from build123d import *

# Parameters (mm, degrees)
BOSS_EXTRUDE1_DEPTH = 7.62
SKETCH2_R           = 7.112
SKETCH2_R_2         = 3.81
BOSS_EXTRUDE2_DEPTH = 12.7
CHAMFER1_SIZE       = 0.508


with BuildPart() as part:
    # Sketch1 → Boss-Extrude1 (new body)
    with BuildSketch(Plane(origin=(0, 0, 0), x_dir=(1, 0, 0), z_dir=(0, 1, 0))):
        Polygon((9.144, 2.794), (7.112, 2.794), (7.112, -2.794), (9.144, -2.794), (9.144, -9.144), (2.794, -9.144), (2.794, -7.112), (-2.794, -7.112), (-2.794, -9.144), (-9.144, -9.144), (-9.144, -2.794), (-7.112, -2.794), (-7.112, 2.794), (-9.144, 2.794), (-9.144, 9.144), (-2.794, 9.144), (-2.794, 7.112), (2.794, 7.112), (2.794, 9.144), (9.144, 9.144), align=None)
    extrude(amount=BOSS_EXTRUDE1_DEPTH)

    # Sketch2 → Boss-Extrude2 (add)
    with BuildSketch(Plane(origin=(0, 7.62, 0), x_dir=(1, 0, 0), z_dir=(0, 1, 0))):
        with Locations(Location((0, 0, 0), (0, 0, 270))):
            Circle(SKETCH2_R)
        with Locations(Location((0, 0, 0), (0, 0, 270))):
            Circle(SKETCH2_R_2, mode=Mode.SUBTRACT)
    extrude(amount=BOSS_EXTRUDE2_DEPTH)

    # Chamfer1
    chamfer1_edges = [part.edges().sort_by_distance(p)[0] for p in [
        (0, 20.32, -3.81),
    ]]
    chamfer(chamfer1_edges, length=CHAMFER1_SIZE)


solid = part.part
Here's how the part is built. I have some questions about the finished solid (model axes, mm). A direction names the side the tool comes from. Coordinates: 2 decimals unless noted, no trailing zeros. Write each loop counter-clockwise with the first axis right and the second up, starting at its lowest first coordinate (ties: lowest second). Pieces come first, ordered by that corner, then holes. Notation, with made-up numbers: (2, 33) - (56, 33) arc R23 cw to (56, 58) - close; hole circle Ø1 at (61, -2). An arc over 180 degrees is marked (long way). Use one line per item in the form item = value.
1) I'm going to push flat-ended pins straight in: P1, Ø3, axis at y = 8.5, z = 4.5, coming from the +X side; P2, Ø2.5, axis at x = -5.5, z = 7, coming from the +Y side; P3, Ø5, axis at x = 6, y = 11.5, coming from the +Z side; P4, Ø10, axis at x = -6, y = 13, coming from the -Z side. Where does each tip first touch, or does it pass through?
Solved:
P1 = 9.14
P2 = 7.62
P3 = 6.19
P4 = -7.04
2) Suppose I cut it at A-A, the plane x = -7.75. Write out the boundary of the cut face in (y, z).
Solved:
outline = (0, -9.14) - (7.62, -9.14) - (7.62, -2.79) - (0, -2.79) - close; (0, 2.79) - (7.62, 2.79) - (7.62, 9.14) - (0, 9.14) - close
3) On a 3-axis mill with a long thin cutter (end or side, diameter ignored), from which of +Z, -Z, +X, -X, +Y, -Y can I reach the whole of each face in a straight line? I mean faces 1 (the flat face through (0, 4, 7.112)), 2 (the flat face through (-7, 7.62, -7)), 3 (the cylindrical face through (-6.943, 13.881, -1.542)). Say none if no direction works.
Solved:
face_1 = +Z, +Y, -Y
face_2 = -Z, -X, +Y
face_3 = +Y
4) Suppose I cut it at B-B, the plane z = 8. Write out the boundary of the cut face in (x, y).
Solved:
outline = (-9.14, 0) - (-2.79, 0) - (-2.79, 7.62) - (-9.14, 7.62) - close; (2.79, 0) - (9.14, 0) - (9.14, 7.62) - (2.79, 7.62) - close
5) Suppose I cut it at C-C, the plane y = 6. Write out the boundary of the cut face in (x, z), plus the area to 3 significant figures.
Solved:
outline = (-9.14, -9.14) - (-2.79, -9.14) - (-2.79, -7.11) - (2.79, -7.11) - (2.79, -9.14) - (9.14, -9.14) - (9.14, -2.79) - (7.11, -2.79) - (7.11, 2.79) - (9.14, 2.79) - (9.14, 9.14) - (2.79, 9.14) - (2.79, 7.11) - (-2.79, 7.11) - (-2.79, 9.14) - (-9.14, 9.14) - (-9.14, 2.79) - (-7.11, 2.79) - (-7.11, -2.79) - (-9.14, -2.79) - close
area = 289 mm2
6) I need wall thicknesses on line 1 (X direction, y = 14.5, z = 0); line 2 (Z direction, x = -7.5, y = 3.25); line 3 (Y direction, x = 2, z = -7). Which ranges of each line are inside material? Lowest first, please.
Solved:
line_1 = -7.11 to -3.81, 3.81 to 7.11
line_2 = -9.14 to -2.79, 2.79 to 9.14
line_3 = 0 to 7.62
7) Suppose I cut it at D-D, the plane z = -5. Write out the boundary of the cut face in (x, y).
Solved:
outline = (-9.14, 0) - (9.14, 0) - (9.14, 7.62) - (5.06, 7.62) - (5.06, 20.32) - (-5.06, 20.32) - (-5.06, 7.62) - (-9.14, 7.62) - close
